```python
from build123d import *

# Parameters (mm, degrees)
ESBO_O1_W                = 12.7
ESBO_O1_H                = 21.6
RESSALTO_EXTRUS_O1_DEPTH = 1.2
ESBO_O2_W                = 2
ESBO_O2_H                = 2
RESSALTO_EXTRUS_O2_DEPTH = 0.5
RESSALTO_EXTRUS_O3_DEPTH = 6


with BuildPart() as part:
    # Esboço1 → Ressalto-extrusão1 (new body)
    with BuildSketch(Plane.XY):
        Rectangle(ESBO_O1_W, ESBO_O1_H)
    extrude(amount=RESSALTO_EXTRUS_O1_DEPTH)

    # Esboço2 → Ressalto-extrusão2 (add)
    with BuildSketch(Plane.XY.offset(1.2)):
        with Locations((0, -2.9)):
            Rectangle(ESBO_O2_W, ESBO_O2_H)
    extrude(amount=RESSALTO_EXTRUS_O2_DEPTH)

    # Esboço3 → Ressalto-extrusão3 (add, symmetric)
    with BuildSketch(Plane(origin=(0, 0, 0), x_dir=(0, 0, -1), z_dir=(1, 0, 0))):
        Polygon((0, 10.3), (1.5, 10.3), (1.5, 13.8), (2.77, 13.8), (2.77, 9.03), (0, 9.03), align=None)
    extrude(amount=RESSALTO_EXTRUS_O3_DEPTH, both=True)


solid = part.part
```
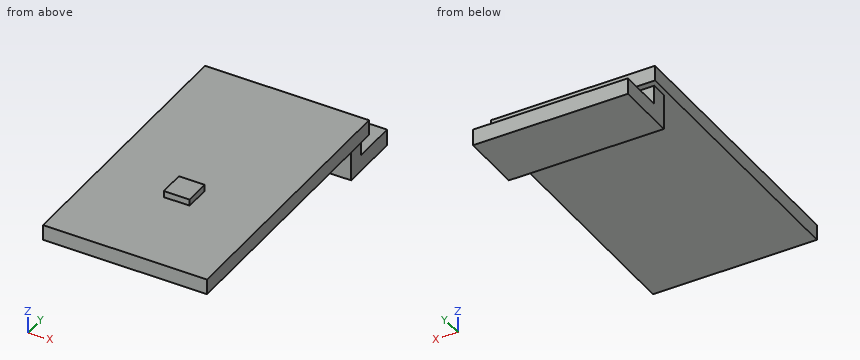
Part model, mm, in its own coordinate system. Give positions to 0.01 mm unless a question says otherwise; leave off trailing zeros. Order: outer loops, then holes, each group sorted by start corner. A loop starts at its lowest first (then second) coordinate and runs counter-clockwise, first axis right, second up. Notation, with made-up numbers: M -33,22.25 L -7,22.25 A19 ccw -7,35.25 Z; hole C 29.25,88.5 d6. An arc over 180 degrees is marked long. Use a Markdown table: item, result. Add a question column.
(1) Saw through at D-D, the plane x = 0.25. Give the cut face in (y, z).
(2) Saw through at A-A, the plane x = -3. Give the cut face in (y, z), and give its area (3 significant figures).
(3) Saw through at B-B, the plane z = 0.5. Give the cut face in (x, y), and give its area (3 significant figures).
(4) Drop flat-ended pins along their axis: P1, Ø0.8, axis at x = -3, z = -0.5, coming from the +Y side; P2, Ø4, axis at x = 4, y = 0, coming from the -Z side; P3, Ø2, axis at x = 2, y = -5, coming from the +Z side; P4, Ø3, axis at x = -3.5, y = 8.5, coming from the -Z side. Give the stop position or say it passes through.
(5) Saw through at C-C, the plane y = 3.25. Give the cut face in (x, z), and give its area (3 significant figures).
(6) Probe line 1 along Y through (x, z) = (-1.25, -1.95); line 2 along Y through (x, z) = (-1.75, -1.05); line 3 along Z through (x, y) = (-1, -9.25). List the from-to ranges inside material, lowest first. Write a range as [from, to].
Answer key:
| question | item | result |
|---|---|---|
| 1 | outline | M -10.8,0 L 9.03,0 L 9.03,-2.77 L 13.8,-2.77 L 13.8,-1.5 L 10.3,-1.5 L 10.3,0 L 10.8,0 L 10.8,1.2 L -1.9,1.2 L -1.9,1.7 L -3.9,1.7 L -3.9,1.2 L -10.8,1.2 Z |
| 2 | outline | M -10.8,0 L 9.03,0 L 9.03,-2.77 L 13.8,-2.77 L 13.8,-1.5 L 10.3,-1.5 L 10.3,0 L 10.8,0 L 10.8,1.2 L -10.8,1.2 Z |
| 2 | area | 33.9 mm^2 |
| 3 | outline | M -6.35,-10.8 L 6.35,-10.8 L 6.35,10.8 L -6.35,10.8 Z |
| 3 | area | 274 mm^2 |
| 4 | P1 | y = 10.3 |
| 4 | P2 | z = 0 |
| 4 | P3 | z = 1.2 |
| 4 | P4 | z = -2.77 |
| 5 | outline | M -6.35,0 L 6.35,0 L 6.35,1.2 L -6.35,1.2 Z |
| 5 | area | 15.2 mm^2 |
| 6 | line 1 | [9.03, 13.8] |
| 6 | line 2 | [9.03, 10.3] |
| 6 | line 3 | [0, 1.2] |
